Could you check a few things on this drawing? It's one solid part, dimensions in mm from its lowest x, y, z. Give positions to 0.01 mm unless a question says otherwise; leave off trailing zeros. Write each loop counter-clockwise with the first axis right and the second up, starting at its lowest first coordinate (ties: lowest second). Pieces come first, ordered by that corner, then holes. Notation, with made-up numbers: M 35,20.25 L 51,20.25 A11 ccw 51,24.25 Z; hole C 17,17 d6. An arc over 180 degrees is marked long. Answer as CSV lines item,"result". Start each with the question number.
Q1. For pin 1 (1.7 mm diameter, centred on x = 8, y = 4.19, fed in from -Z), with a flat end and sliding along its axis, tell me the tip position at first contact or that it passes through.
Q2. Suppose I cut it at C-C (z = 0.7). Write out the boundary of the cut face in (x, y), then the cut area to 3 significant figures.
Q3. Suppose I cut it at D-D (y = 7.75). Write out the boundary of the cut face in (x, z).
Q4. Suppose I cut it at A-A (x = 8). Write out the boundary of the cut face in (y, z), then the cut area to 3 significant figures.
Q5. Thinking about a two-plate mould opening in Y: for the marked faces 1, 2, 3 and 4, which applies, +Y half, -Y half, draft (parallel to the pull), parting line (faces both ways), or undercut?
Q6. If I drill on line 1 along Y through (x, z) = (8, 0.8); line 2 along X through (y, z) = (4.25, 0.7); line 3 along X through (y, z) = (4.75, 0.8), over which ranges is the centre line in solid material (lowest first)?
Q7. Suppose I cut it at B-B (y = 3.5). Write out the boundary of the cut face in (x, z).
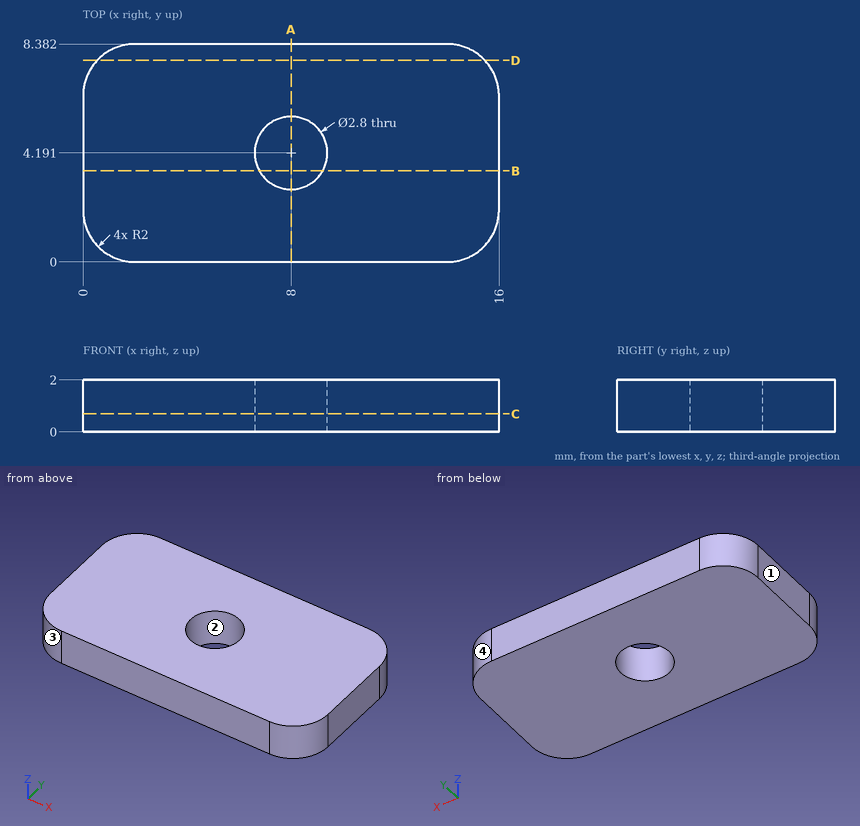
Resolved:
1,pin 1,"through"
2,outline,"M 0,2 A2 ccw 2,0 L 14,0 A2 ccw 16,2 L 16,6.38 A2 ccw 14,8.38 L 2,8.38 A2 ccw 0,6.38 Z; hole C 8,4.19 d2.8"
2,area,"125 mm^2"
3,outline,"M 0.54,0 L 15.46,0 L 15.46,2 L 0.54,2 Z"
4,outline,"M 0,0 L 2.79,0 L 2.79,2 L 0,2 Z; M 5.59,0 L 8.38,0 L 8.38,2 L 5.59,2 Z"
4,area,"11.2 mm^2"
5,face 1,"draft"
5,face 2,"undercut"
5,face 3,"-Y half"
5,face 4,"+Y half"
6,line 1,"0 to 2.79, 5.59 to 8.38"
6,line 2,"0 to 6.6, 9.4 to 16"
6,line 3,"0 to 6.72, 9.28 to 16"
7,outline,"M 0,0 L 6.78,0 L 6.78,2 L 0,2 Z; M 9.22,0 L 16,0 L 16,2 L 9.22,2 Z"
